```python
from build123d import *

# Parameters (mm, degrees)
F0_W     = 24.341667
F0_H     = 19.226389
F0_W_2   = 10.348033
F0_H_2   = 10.113077
F1_DEPTH = 5
F2_R     = 4
F3_R     = 9
F4_R     = 0.5
F5_W     = 85
F5_H     = 130
F6_DEPTH = 6
F7_R     = 4
F8_R     = 1.5


with BuildPart() as f1:
    # F0 (on Top) → F1 (new body)
    with BuildSketch(Plane.XY):
        Polygon((-31.867478, -38.717533), (-38.629167, -38.717533), (-38.629167, -57.532578), (-31.867478, -57.532578), (-31.867478, -53.181422), (-27.693055, -50.182811), (-22.342478, -57.532578), (-14.404978, -57.532578), (-22.577778, -45.655611), (-14.816667, -38.717533), (-23.048033, -38.717533), (-31.867478, -46.831422), align=None)
        Polygon((-5.350405, -38.717533), (-11.935533, -38.717533), (-11.935533, -57.943922), (-5.703183, -57.885356), (-5.526794, -50.8298), (4.027317, -50.91765), (3.939467, -57.943922), (10.583333, -57.943922), (10.583333, -38.717533), (3.880556, -38.717533), (3.880556, -46.0673), (-5.350405, -46.0673), align=None)
        Polygon((-14.875405, 5.085994), (-37.394272, -34.660244), (-15.933567, -34.954111), (-8.231367, -22.077722), (-0.6761, -34.601333), (6.702778, -21.783856), (13.934722, -34.954111), (35.748378, -34.954111), (13.523378, 5.321639), (10.818633, 0.708828), (-0.528994, 57.943922), (-12.347222, 1.704805), align=None)
        Polygon((-18.403183, -30.661178), (-30.456539, -30.661178), (-14.640278, -2.850644), (-10.289294, -9.729811), (-0.823033, 37.366022), (8.760533, -10.1415), (13.111689, -2.615344), (28.516089, -30.661178), (16.227778, -30.661178), (6.5853, -13.669278), (-0.587905, -27.074489), (-8.231539, -13.375066), align=None, mode=Mode.SUBTRACT)
        with Locations((26.458333, -48.330727)):
            Rectangle(F0_W, F0_H)
        with Locations((26.223205, -48.594794)):
            Rectangle(F0_W_2, F0_H_2, mode=Mode.SUBTRACT)
    extrude(amount=F1_DEPTH)

    # F2
    f2_edges = [f1.edges().sort_by_distance(p)[0] for p in [
        (31.397222, -43.538256, 2.5),
        (31.397222, -53.651333, 2.5),
    ]]
    fillet(f2_edges, radius=F2_R)

    # F3
    f3_edges = [f1.edges().sort_by_distance(p)[0] for p in [
        (38.629167, -57.943922, 2.5),
        (38.629167, -38.717533, 2.5),
    ]]
    fillet(f3_edges, radius=F3_R)

    # F4
    f4_edges = [f1.edges().sort_by_distance(p)[0] for p in [
        (-38.629167, -38.717533, 2.5),
        (-31.867478, -38.717533, 2.5),
        (-23.048033, -38.717533, 2.5),
        (-14.816667, -38.717533, 2.5),
        (-31.867478, -46.831422, 2.5),
        (-22.577778, -45.655611, 2.5),
        (-14.404978, -57.532578, 2.5),
        (-22.342478, -57.532578, 2.5),
        (-27.693055, -50.182811, 2.5),
        (-31.867478, -53.181422, 2.5),
        (-31.867478, -57.532578, 2.5),
        (-38.629167, -57.532578, 2.5),
        (-11.935533, -57.943922, 2.5),
        (-5.703183, -57.885356, 2.5),
        (4.027317, -50.91765, 2.5),
        (3.939467, -57.943922, 2.5),
        (10.583333, -57.943922, 2.5),
        (14.2875, -57.943922, 2.5),
        (14.2875, -38.717533, 2.5),
        (13.934722, -34.954111, 2.5),
        (-0.6761, -34.601333, 2.5),
        (-37.394272, -34.660244, 2.5),
        (-15.933567, -34.954111, 2.5),
        (-8.231367, -22.077722, 2.5),
        (-5.526794, -50.8298, 2.5),
        (21.049189, -53.651333, 2.5),
        (21.049189, -43.538256, 2.5),
        (10.583333, -38.717533, 2.5),
        (-5.350405, -38.717533, 2.5),
        (-5.350405, -46.0673, 2.5),
        (-11.935533, -38.717533, 2.5),
        (3.880556, -46.0673, 2.5),
        (-0.587905, -27.074489, 2.5),
        (6.5853, -13.669278, 2.5),
        (16.227778, -30.661178, 2.5),
        (-8.231539, -13.375066, 2.5),
        (-18.403183, -30.661178, 2.5),
        (-30.456539, -30.661178, 2.5),
        (-14.875405, 5.085994, 2.5),
        (-10.289294, -9.729811, 2.5),
        (8.760533, -10.1415, 2.5),
        (28.516089, -30.661178, 2.5),
        (13.111689, -2.615344, 2.5),
        (13.523378, 5.321639, 2.5),
        (-0.823033, 37.366022, 2.5),
        (-0.528994, 57.943922, 2.5),
        (-14.640278, -2.850644, 2.5),
    ]]
    fillet(f4_edges, radius=F4_R)

    # F5 (on face) → F6 (join)
    with BuildSketch(Plane(origin=(0, 0, 0), x_dir=(1, 0, 0), z_dir=(0, 0, -1))):
        Rectangle(F5_W, F5_H)
    extrude(amount=F6_DEPTH)

    # F7
    f7_edges = [f1.edges().sort_by_distance(p)[0] for p in [
        (42.5, -65, -3),
        (42.5, 65, -3),
        (-42.5, 65, -3),
        (-42.5, -65, -3),
    ]]
    fillet(f7_edges, radius=F7_R)

    # F8
    f8_edges = [f1.edges().sort_by_distance(p)[0] for p in [
        (0, -65, 0),
    ]]
    fillet(f8_edges, radius=F8_R)


solid = f1.part
```
The listing builds one solid part. Answer for the finished solid, in the listing's coordinates (mm). A direction names the side the tool comes from. Give positions to 0.01 mm unless a question says otherwise; leave off trailing zeros. Write each loop counter-clockwise with the first axis right and the second up, starting at its lowest first coordinate (ties: lowest second). Pieces come first, ordered by that corner, then holes. Notation, with made-up numbers: (33, 51.5) - (71, 51.5) arc R13 cw to (71, 58.5) - close; hole circle Ø10 at (40.5, -31.5). An arc over 180 degrees is marked (long way). Use one line per item in the form item = value. Start each with the question number.
1) Find section D-D on x = -26. Determine the outline of the cut face in (y, z), plus the area to 3 significant figures.
2) The mould has two halves that part along X. Classify faces 6 (the face through (22, -30.661, 2)), 7 (the face through (-41.359, 63.797, -3.781)), 8 (the face through (35.92, -41.28, 2.54)): pulls with the +X half, pulls with the -X half, needs draft (parallel to the pull), parting line crosses it, or undercut.
3) Consider line 1 along X through (y, z) = (-6, 2.75); line 2 along Z through (x, y) = (-14, -5.5); line 3 along Y through (x, z) = (-37, -1.25). Determine where each line is inside the solid, lowest interval first. Write a range as from..to.
4) Find section C-C on y = -10.5. Determine the outline of the cut face in (x, z).
5) Find section A-A on z = 3.75. Count the separate pieces of the cut face and the enclosed holes in it, plus the area to 3 significant figures.
6) A tool of negligible diameter and unlimited length cuts with its end or side. For faces 1 (the face through (-38.629, -48, 2)), 2 (the face through (25, -34.954, 2)), 3 (the face through (-11.936, -48, 2)), 4 (the face through (3.176, -27.91, 2.465)), 5 (the face through (42.5, 1, -4)), from which of +Z, -Z, +X, -X, +Y, -Y can it reach the whole face along a straight path? Write none if from no direction.
7) Find section B-B on x = 34.5. Determine the outline of the cut face in (y, z), plus the area to 3 significant figures.
8) Flat-ended cylindrical pins translate along their axes: pin 1 Ø1 at (x, z) = (25.5, -0.5) entering from +Y; pin 2 Ø4 at (x, z) = (6.5, 3.5) entering from -Y; pin 3 Ø4 at (x, y) = (-27.5, 38) entering from +Z. Find the tip coordinate at first contact, or state that the pin passes through.
Geometry results:
q1.outline = (-65, -6) - (65, -6) - (65, -1.5) arc R1.5 ccw to (63.5, 0) - (-14.55, 0) - (-14.55, 5) - (-22.83, 5) - (-22.83, 0) - (-30.66, 0) - (-30.66, 5) - (-34.82, 5) - (-34.82, 0) - (-41.43, 0) - (-41.43, 5) - (-52.51, 5) - (-52.51, 0) - (-63.5, 0) arc R1.5 ccw to (-65, -1.5) - close
q1.area = 897 mm2
q2.face_6 = undercut
q2.face_7 = pulls with the -X half
q2.face_8 = pulls with the +X half
q3.line_1 = -21.16..-16.43, -12.65..-9.54, 7.93..11.15, 14.97..19.77
q3.line_2 = -6..0
q3.line_3 = -64.98..64.98
q4.outline = (-42.5, -6) - (42.5, -6) - (42.5, -1.5) arc R1.5 ccw to (41, 0) - (22.25, 0) - (22.25, 5) - (17.44, 5) - (17.44, 0) - (-18.99, 0) - (-18.99, 5) - (-23.71, 5) - (-23.71, 0) - (-41, 0) arc R1.5 ccw to (-42.5, -1.5) - close
q5.separate_pieces = 4
q5.enclosed_holes = 2
q5.area = 2,160 mm2
q6.face_1 = +Z, -X, +Y, -Y
q6.face_2 = +Z, +X, -X
q6.face_3 = +Z, -Y
q6.face_4 = +Z
q6.face_5 = +Z, -Z, +X, +Y, -Y
q7.outline = (-65, -6) - (65, -6) - (65, -1.5) arc R1.5 ccw to (63.5, 0) - (-32.69, 0) - (-32.69, 5) - (-34.95, 5) - (-34.95, 0) - (-40.15, 0) - (-40.15, 5) - (-56.51, 5) - (-56.51, 0) - (-63.5, 0) arc R1.5 ccw to (-65, -1.5) - close
q7.area = 872 mm2
q8.pin_1 = 64.91
q8.pin_2 = -57.94
q8.pin_3 = 0
